Here's the drawing with two shaded views (mm, measured from the low corner). I have some questions. A direction names the side the tool comes from. Give positions to 0.01 mm unless a question says otherwise; leave off trailing zeros. Loops run counter-clockwise (first coordinate to the right, second up) from the corner with the lowest first, then second, coordinate; pieces in that order, holes last. Notation, with made-up numbers: M 3.5,-38 L 19.5,-38 A15 ccw 19.5,-24 Z; hole C -16,1 d6. An arc over 180 degrees is marked long. Use CSV: the item, a comma, the result in double quotes.
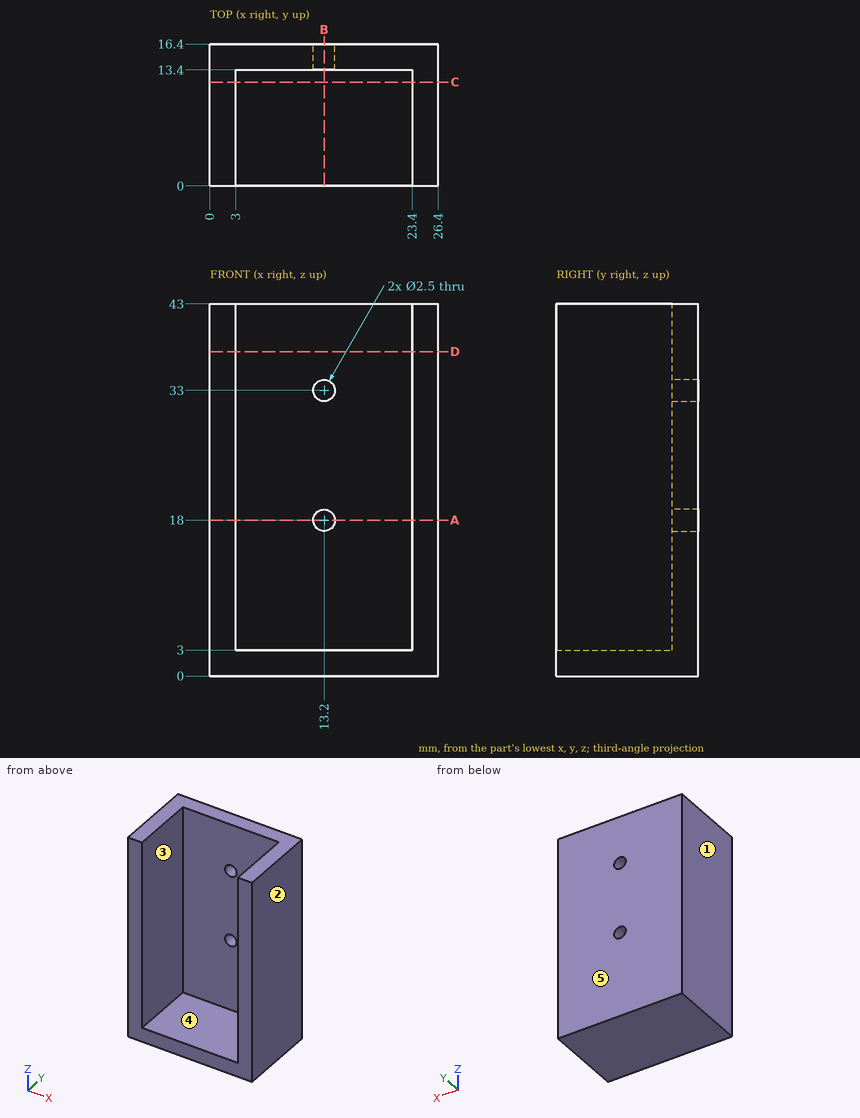
1. Please list where these lines run through material, in increasing order: line 1 (X direction, y = 14.55, z = 33); line 2 (X direction, y = 2.75, z = 10); line 3 (Y direction, x = 16.75, z = 23.5).
Outcome:
line 1,"0 to 11.95, 14.45 to 26.4"
line 2,"0 to 3, 23.4 to 26.4"
line 3,"13.4 to 16.4"
2. I want a section at A-A, the plane z = 18. List the corners of the cut face in (x, y) for me.
Outcome:
outline,"M 0,0 L 3,0 L 3,13.4 L 11.95,13.4 L 11.95,16.4 L 0,16.4 Z; M 14.45,13.4 L 23.4,13.4 L 23.4,0 L 26.4,0 L 26.4,16.4 L 14.45,16.4 Z"
3. I want a section at C-C, the plane y = 12. List the corners of the cut face in (x, z) for me.
Outcome:
outline,"M 0,0 L 26.4,0 L 26.4,43 L 23.4,43 L 23.4,3 L 3,3 L 3,43 L 0,43 Z"
4. Which directions (+Z, -Z, +X, -X, +Y, -Y) give clear straight access to the entire face, cutting with the end or side of a thin tool? Please do the marked faces 4 and 5.
Outcome:
face 4,"+Z, -Y"
face 5,"+Z, -Z, +X, -X, +Y"
5. If we mould it in two halves opening along X, with no side actions, what happens to the marked faces 1, 2 and 3? For each: +X half, -X half, draft (parallel to the pull), parting line (faces both ways), or undercut.
Outcome:
face 1,"-X half"
face 2,"+X half"
face 3,"undercut"
6. I want a section at D-D, the plane z = 37.5. List the corners of the cut face in (x, y) for me, then the cut area to 3 significant figures.
Outcome:
outline,"M 0,0 L 3,0 L 3,13.4 L 23.4,13.4 L 23.4,0 L 26.4,0 L 26.4,16.4 L 0,16.4 Z"
area,"160 mm2"
7. I'm going to push flat-ended pins straight in: pin 1 Ø8 at (x, y) = (6.5, 6.5) entering from +Z; pin 2 Ø6 at (x, y) = (7, 8.5) entering from +Z; pin 3 Ø10 at (x, z) = (11, 16) entering from -Y. Where does each tip first touch, or does it pass through?
Outcome:
pin 1,"z = 43"
pin 2,"z = 3"
pin 3,"y = 13.4"
8. I want a section at B-B, the plane x = 13.2. List the corners of the cut face in (y, z) for me, then the cut area to 3 significant figures.
Outcome:
outline,"M 0,0 L 16.4,0 L 16.4,16.75 L 13.4,16.75 L 13.4,3 L 0,3 Z; M 13.4,19.25 L 16.4,19.25 L 16.4,31.75 L 13.4,31.75 Z; M 13.4,34.25 L 16.4,34.25 L 16.4,43 L 13.4,43 Z"
area,"154 mm2"
